Autodesk Inventor part; units mm, degrees
ref_plane "YZ Plane" through (0, 0, 0) normal (1, 0, 0) x (0, 1, 0)
ref_plane "XZ Plane" through (0, 0, 0) normal (0, 1, 0) x (-1, 0, 0)
ref_plane "XY Plane" through (0, 0, 0) normal (0, 0, 1) x (1, 0, 0)
sketch "Náčrt1" plane through (0, 0, 0) normal (0, 0, 1) x (1, 0, 0)
  line L0 (0, 0) -> (-90, 0)
  line L1 (-90, 0) -> (-90, 30)
  line L2 (-45, 0) -> (-45, 128.8279) construction
  line L3 (-45, 100) -> (-65, 100)
  line L4 (-90, 30) -> (-65, 100)
  line L5 (0, 0) -> (0, 30)
  line L6 (-45, 100) -> (-25, 100)
  line L7 (0, 30) -> (-25, 100)
  circle A0 centre (-45, 80) radius 10
  circle A1 centre (-75, 15) radius 6.5
  circle A2 centre (-75, 15) radius 10
  circle A3 centre (-15, 15) radius 6.5
  circle A4 centre (-15, 15) radius 10
  dimension "d0" = 90
  dimension "d1" = 30
  dimension "d4" = 20
  dimension "d5" = 100
  dimension "d6" = 20
  dimension "d7" = 80
  dimension "d8" = 13
  dimension "d10" = 15
  dimension "d11" = 20
  dimension "d12" = 15
extrude "Vysunutí1" add sketch "Náčrt1" along normal blind 30 contours L0 L1 L4 L3 L6 L7 L5
sketch "Náčrt2" plane through (0, 0, 0) normal (0, 0, 1) x (1, 0, 0)
  circle A0 centre (-15, 15) radius 10
  circle A1 centre (-75, 15) radius 10
  circle A2 centre (-75, 15) radius 6.5
  circle A3 centre (-15, 15) radius 6.5
  point P0 (0, 0)
  dimension "d15" = 13
  dimension "d16" = 13
extrude "Vysunutí2" add sketch "Náčrt2" along normal blind 18
sketch "Náčrt3" plane through (-90, 0, 0) normal (-1, 0, 0) x (0, 0, 1)
  line L0 (0, 30) -> (30, 30) construction
  line L1 (15, 30) -> (15, 100) construction
  line L2 (0, 100) -> (30, 100) construction
  line L3 (15, 50) -> (22, 50)
  line L4 (22, 50) -> (22, 100)
  line L5 (22, 100) -> (15, 100)
  line L6 (30, 100) -> (0, 100) construction
  line L7 (15, 50) -> (8, 50)
  line L8 (8, 50) -> (8, 100)
  line L9 (8, 100) -> (15, 100)
  point P0 (0, 0)
  dimension "d19" = 7
  dimension "d20" = 50
extrude "Vysunutí3" cut sketch "Náčrt3" against normal through all
properties part number "Součást9"
Geometry check sheet. Reference: the model listing, model coordinates, mm. A direction names the side the tool comes from. Round coordinates to 2 decimals unless told otherwise and drop trailing zeros. Order: outer loops, then holes, each group sorted by start corner. A loop starts at its lowest first (then second) coordinate and runs counter-clockwise, first axis right, second up. Notation, with made-up numbers: (-28, 43.5) - (14, 43.5) arc R19 cw to (14, 63.5) - close; hole circle Ø5 at (23, 87). An arc over 180 degrees is marked (long way). Use a Markdown table: item, result. Add a question column.
1) Section check D-D (z = 4.25). Record the cut outline in (x, y).
2) Mould release check, pull along Y, two halves, no side actions. Record for faces 4 (the flat face through (-46, 69, 22)), 5 (the flat face through (-45, 100, 4)), 6 (the cylindrical face through (-46.302, 70.085, 25.944)): released by +Y, released by -Y, zero draft, split by the parting line, or undercut.
3) Section check B-B (y = 15). Record the cut outline in (x, z).
4) Thickness scan on line 1 along Y through (x, z) = (-15, 8.5); line 2 along Z through (x, y) = (-23, 63.5); line 3 along Y through (x, z) = (-45, 26.25). Record the ranges inside material, lowest first.
5) Section check A-A (x = -45). Record the cut outline in (y, z).
6) Set-up check for faces 1 (the flat face through (-90, 15, 15)), 2 (the flat face through (-46, 69, 8)), 3 (the cylindrical face through (-5.46, 12, 23.92)): record each of +Z, -Z, +X, -X, +Y, -Y from which the full face is reachable in a straight line by a thin tool's end or side.
7) Section check C-C (x = -15). Record the cut outline in (y, z), then the cut area to 3 significant figures.
8) Gauge pin test, flat ends, axial feed: P1, Ø1, axis at y = 39, z = 4.5, coming from the -X side; P2, Ø23, axis at x = -45, y = 80, coming from the +Z side; P3, Ø4, axis at x = -51, z = 17.5, coming from the +Y side; P4, Ø10, axis at y = 42, z = 23, coming from the -X side. Record the tip position at first contact, or that the pin passes through.
Established:
| question | item | result |
|---|---|---|
| 1 | outline | (-90, 0) - (0, 0) - (0, 30) - (-25, 100) - (-65, 100) - (-90, 30) - close; hole circle Ø13 at (-75, 15); hole circle Ø20 at (-45, 80); hole circle Ø13 at (-15, 15) |
| 2 | face 4 | zero draft |
| 2 | face 5 | released by +Y |
| 2 | face 6 | undercut |
| 3 | outline | (-90, 0) - (-81.5, 0) - (-81.5, 18) - (-85, 18) - (-85, 30) - (-90, 30) - close; (-68.5, 0) - (-21.5, 0) - (-21.5, 18) - (-25, 18) - (-25, 30) - (-65, 30) - (-65, 18) - (-68.5, 18) - close; (-8.5, 0) - (0, 0) - (0, 30) - (-5, 30) - (-5, 18) - (-8.5, 18) - close |
| 4 | line 1 | 0 to 8.5, 21.5 to 50 |
| 4 | line 2 | 0 to 8, 22 to 30 |
| 4 | line 3 | 0 to 70, 90 to 100 |
| 5 | outline | (0, 0) - (70, 0) - (70, 8) - (50, 8) - (50, 22) - (70, 22) - (70, 30) - (0, 30) - close; (90, 0) - (100, 0) - (100, 8) - (90, 8) - close; (90, 22) - (100, 22) - (100, 30) - (90, 30) - close |
| 6 | face 1 | +Z, -Z, -X, +Y, -Y |
| 6 | face 2 | +X, -X, +Y |
| 6 | face 3 | +Z |
| 7 | outline | (0, 0) - (8.5, 0) - (8.5, 18) - (5, 18) - (5, 30) - (0, 30) - close; (21.5, 0) - (72, 0) - (72, 8) - (50, 8) - (50, 22) - (72, 22) - (72, 30) - (25, 30) - (25, 18) - (21.5, 18) - close |
| 7 | area | 1,380 mm2 |
| 8 | P1 | x = -86.96 |
| 8 | P2 | z = 30 |
| 8 | P3 | y = 50 |
| 8 | P4 | x = -87.5 |
